Design review of the part built by this model. Coordinates are the model's own, in mm. A direction names the side the tool comes from. Give positions to 0.01 mm unless a question says otherwise; leave off trailing zeros. Order: outer loops, then holes, each group sorted by start corner. A loop starts at its lowest first (then second) coordinate and runs counter-clockwise, first axis right, second up. Notation, with made-up numbers: (-21.5, -36.5) -> (5.5, -36.5) arc R24 cw to (5.5, -3.5) -> close; hole circle Ø5 at (-2.5, -28). An arc over 180 degrees is marked (long way). Use a Markdown table: item, result. Add a question column.
```python
from build123d import *

# Parameters (mm, degrees)
SKETCH1_R             = 2.4
BOSS_EXTRUDE1_DEPTH   = 4.2
BOSS_EXTRUDE1_2_DEPTH = 4.2
BOSS_EXTRUDE1_3_DEPTH = 4.2
SKETCH2_W             = 14.663185534
SKETCH2_H             = 1.5
BOSS_EXTRUDE2_DEPTH   = 0.8
SKETCH3_R             = 3.25
BOSS_EXTRUDE3_DEPTH   = 1.5


with BuildPart() as part:
    # Sketch1 → Boss-Extrude1 (new body)
    with BuildSketch(Plane.XY):
        with Locations((-7.5, 0)):
            Circle(SKETCH1_R)
    extrude(amount=BOSS_EXTRUDE1_DEPTH)



with BuildPart() as body_2:
    # Sketch1 → Boss-Extrude1 2 (new body)
    with BuildSketch(Plane.XY):
        Circle(SKETCH1_R)
    extrude(amount=BOSS_EXTRUDE1_2_DEPTH)


with BuildPart() as body_3:
    # Sketch1 → Boss-Extrude1 3 (new body)
    with BuildSketch(Plane.XY):
        with Locations((7.5, 0)):
            Circle(SKETCH1_R)
    extrude(amount=BOSS_EXTRUDE1_3_DEPTH)


with BuildPart() as part_1:
    add(part.part)

    add(body_2.part)  # Boss-Extrude2 merges body 2

    add(body_3.part)  # Boss-Extrude2 merges body 3
    # Sketch2 → Boss-Extrude2 (add)
    with BuildSketch(Plane(origin=(0, 0, 0), x_dir=(-1, 0, 0), z_dir=(0, 0, -1))):
        Rectangle(SKETCH2_W, SKETCH2_H)
    extrude(amount=-BOSS_EXTRUDE2_DEPTH)

    # Sketch3 → Boss-Extrude3 (add)
    with BuildSketch(Plane(origin=(0, 0, 0), x_dir=(-1, 0, 0), z_dir=(0, 0, -1))):
        Circle(SKETCH3_R)
        with Locations((7.5, 0)):
            Circle(SKETCH3_R)
        with Locations((-7.5, 0)):
            Circle(SKETCH3_R)
    extrude(amount=-BOSS_EXTRUDE3_DEPTH)


solid = part_1.part
```
1) Add section B-B (y = 2). Give the boundary of the cut face in (x, z), then the cut area to 3 significant figures.
2) For L1, parallel to X at y = 1.75, z = 1.1; L2, parallel to X at y = 1.75, z = 3; L3, parallel to Z at x = 5, y = 0.25, list the stretches that pass through material, from the lowest coordinate up. Write a range as [from, to].
3) Add section C-C (x = 0). Give the boundary of the cut face in (y, z).
4) Add section A-A (z = 0.4). Give the boundary of the cut face in (x, y), then the cut area to 3 significant figures.
5) The part is to be moulded in two halves that separate along X. For faces 1 (the flat face through (0, 0, 4.2)), 2 (the flat face through (-4, 0, 0.8)), say which applies: +X half, -X half, draft (parallel to the pull), parting line (faces both ways), or undercut.
6) Machinability: for faces 3 (the cylindrical face through (9.717, -0.919, 2.831)), 4 (the flat face through (0, 0, 0)), which of the approach directions +Z, -Z, +X, -X, +Y, -Y give a long, thin tool a straight path to every point of the face, cutting with its end or side? Answer none if there is none.
7) Insertion check: pin 1 (2 mm diameter, centred on y = -0.5, z = 3, fed in from +X); pin 2 (0.9 mm diameter, centred on x = -4, y = 0, fed in from +Z); pin 3 (0.6 mm diameter, centred on x = -3.5, z = 0.5, fed in from -Y). Each pin has a flat end and moves straight along its axis. Give the tip position at first contact, or say it passes through.
8) Add section D-D (y = 0). Give the boundary of the cut face in (x, z), then the cut area to 3 significant figures.
Worked answers:
| question | item | result |
|---|---|---|
| 1 | outline | (-10.06, 0) -> (-4.94, 0) -> (-4.94, 1.5) -> (-6.17, 1.5) -> (-6.17, 4.2) -> (-8.83, 4.2) -> (-8.83, 1.5) -> (-10.06, 1.5) -> close; (-2.56, 0) -> (2.56, 0) -> (2.56, 1.5) -> (1.33, 1.5) -> (1.33, 4.2) -> (-1.33, 4.2) -> (-1.33, 1.5) -> (-2.56, 1.5) -> close; (4.94, 0) -> (10.06, 0) -> (10.06, 1.5) -> (8.83, 1.5) -> (8.83, 4.2) -> (6.17, 4.2) -> (6.17, 1.5) -> (4.94, 1.5) -> close |
| 1 | area | 44.5 mm^2 |
| 2 | L1 | [-10.24, -4.76], [-2.74, 2.74], [4.76, 10.24] |
| 2 | L2 | [-9.14, -5.86], [-1.64, 1.64], [5.86, 9.14] |
| 2 | L3 | [0, 1.5] |
| 3 | outline | (-3.25, 0) -> (3.25, 0) -> (3.25, 1.5) -> (2.4, 1.5) -> (2.4, 4.2) -> (-2.4, 4.2) -> (-2.4, 1.5) -> (-3.25, 1.5) -> close |
| 4 | outline | (-4.34, -0.75) -> (-3.16, -0.75) arc R3.25 ccw to (3.16, -0.75) -> (4.34, -0.75) arc R3.25 ccw (long way) to (4.34, 0.75) -> (3.16, 0.75) arc R3.25 ccw to (-3.16, 0.75) -> (-4.34, 0.75) arc R3.25 ccw (long way) to start |
| 4 | area | 103 mm^2 |
| 5 | face 1 | draft |
| 5 | face 2 | undercut |
| 6 | face 3 | +Z |
| 6 | face 4 | -Z, +X, -X, +Y, -Y |
| 7 | pin 1 | x = 9.9 |
| 7 | pin 2 | z = 1.5 |
| 7 | pin 3 | y = -0.75 |
| 8 | outline | (-10.75, 0) -> (10.75, 0) -> (10.75, 1.5) -> (9.9, 1.5) -> (9.9, 4.2) -> (5.1, 4.2) -> (5.1, 1.5) -> (4.25, 1.5) -> (4.25, 0.8) -> (3.25, 0.8) -> (3.25, 1.5) -> (2.4, 1.5) -> (2.4, 4.2) -> (-2.4, 4.2) -> (-2.4, 1.5) -> (-3.25, 1.5) -> (-3.25, 0.8) -> (-4.25, 0.8) -> (-4.25, 1.5) -> (-5.1, 1.5) -> (-5.1, 4.2) -> (-9.9, 4.2) -> (-9.9, 1.5) -> (-10.75, 1.5) -> close |
| 8 | area | 69.7 mm^2 |
